Job drawing, mm, ordinate dimensions from the low corner. One solid piece. A direction names the side the tool comes from. Round coordinates to 2 decimals unless told otherwise and drop trailing zeros. Write each loop counter-clockwise with the first axis right and the second up, starting at its lowest first coordinate (ties: lowest second). Pieces come first, ordered by that corner, then holes.
1) Saw through at B-B on z = 0.65. Write the cut outline in (x, y), and give its area (3 significant figures).
2) Pull direction X, two halves, no side cores. Call the marked faces 4, 5, 6 and 7: +X half, -X half, draft (parallel to the pull), parting line (faces both ways), or undercut.
3) Flat gauge pins, fed straight in: pin 1 (1.3 mm diameter, centred on x = 19.5, y = 4, fed in from -Z) (1 decimal); pin 2 (0.8 mm diameter, centred on x = 12, y = 4.5, fed in from -Z) (3 decimals). Where does each tip first touch, or does it go through?
4) Saw through at C-C on z = 1.9. Count the separate pieces of the cut face and the enclosed holes in it, and give its area (3 significant figures).
5) Which spindle directions (+Z, -Z, +X, -X, +Y, -Y) get a long thin tool onto all of the face, cutting with end or side? Do the marked faces 1, 2 and 3. Say none if no direction does.
6) Saw through at D-D on y = 2.25. Write the cut outline in (x, z) (1 decimal).
7) Drill centre lines: L1, parallel to X at y = 6, z = 0.95; L2, parallel to Y at x = 10, z = 1.15; L3, parallel to X at y = 3.5, z = 3.7 (1 decimal). Where is each one in solid material? Low to high.
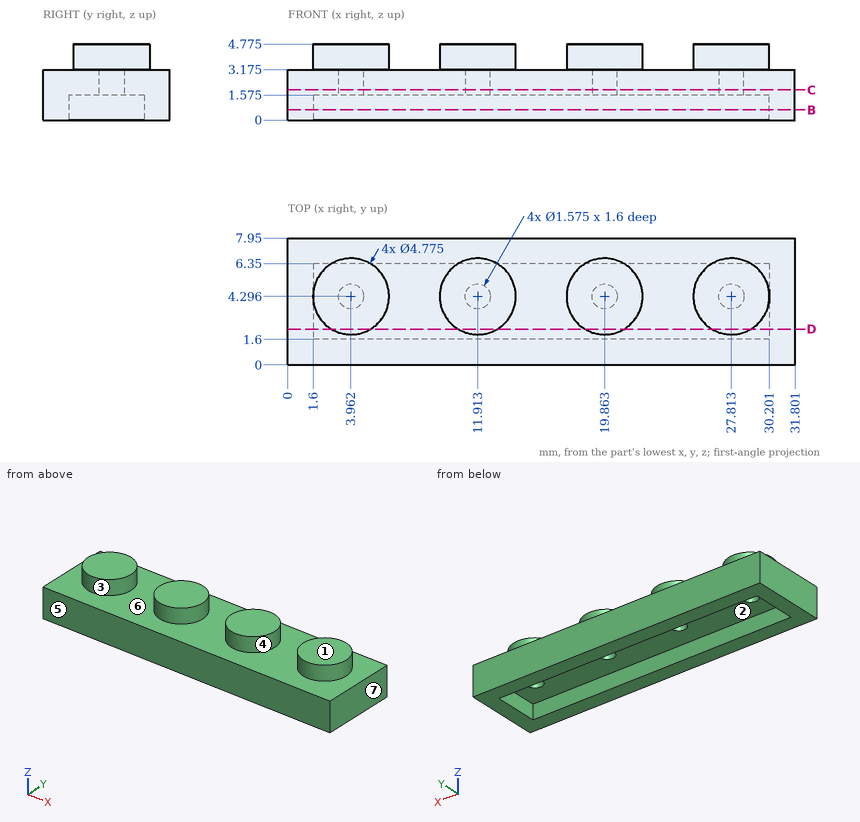
Completed:
1. outline: (0, 0) - (31.8, 0) - (31.8, 7.95) - (0, 7.95) - close; hole (1.6, 1.6) - (30.2, 1.6) - (30.2, 6.35) - (1.6, 6.35) - close
1. area: 117 mm2
2. face 4: undercut
2. face 5: draft
2. face 6: undercut
2. face 7: +X half
3. pin 1: stops at z = 1.6
3. pin 2: stops at z = 3.175
4. separate pieces: 1
4. enclosed holes: 4
4. area: 245 mm2
5. face 1: +Z, +X, -X, +Y, -Y
5. face 2: -Z
5. face 3: +Z
6. outline: (0, 0) - (1.6, 0) - (1.6, 1.6) - (30.2, 1.6) - (30.2, 0) - (31.8, 0) - (31.8, 3.2) - (29, 3.2) - (29, 4.8) - (26.6, 4.8) - (26.6, 3.2) - (21.1, 3.2) - (21.1, 4.8) - (18.6, 4.8) - (18.6, 3.2) - (13.1, 3.2) - (13.1, 4.8) - (10.7, 4.8) - (10.7, 3.2) - (5.2, 3.2) - (5.2, 4.8) - (2.7, 4.8) - (2.7, 3.2) - (0, 3.2) - close
7. L1: x = 0 to 1.6, 30.2 to 31.8
7. L2: y = 0 to 1.6, 6.35 to 7.95
7. L3: x = 1.7 to 6.2, 9.7 to 14.2, 17.6 to 22.1, 25.6 to 30.1
